Design review of the part built by this model. Coordinates are the model's own, in mm. Face numbers are marked on the shaded views. A direction names the side the tool comes from. Round coordinates to 2 decimals unless told otherwise and drop trailing zeros. Loops run counter-clockwise (first coordinate to the right, second up) from the corner with the lowest first, then second, coordinate; pieces in that order, holes last. Notation, with made-up numbers: (44.5, -8) -> (63.5, -8) arc R17 cw to (63.5, 20) -> close; hole circle Ø7 at (54.5, 44). An arc over 180 degrees is marked (long way). Answer as CSV lines item,"result". Start each with the question number.
(1) Take a section at B-B, the plane z = 95. Write out the cut boundary in (x, y), and give its area (3 significant figures).
(2) Take a section at C-C, the plane y = 79.5. Write out the cut boundary in (x, z), and give its area (3 significant figures).
(3) For P1, Ø5, axis at x = 25, z = -28.5, coming from the -Y side; P2, Ø6, axis at y = 97.5, z = 87, coming from the -X side, all flat-tipped, find the tip position at first contact; note any pin that passes through.
(4) Take a section at A-A, the plane x = -86. Write out the cut boundary in (y, z).
(5) To check wall thickness, follow line 1 (X direction, y = 5.5, z = -109.5); line 2 (X direction, y = -208.5, z = 106.5); line 3 (Z direction, x = -41, y = -149.5). State the ranges of each line that lie inside material, in increasing order. Write a range as from..to.
(6) Machinability: for the marked faces 4, 5 and 6, which of the approach directions +Z, -Z, +X, -X, +Y, -Y give a long, thin tool a straight path to every point of the face, cutting with its end or side? Answer none if there is none.
(7) Draft analysis for pull direction Z (two halves, no side actions). For the marked faces 1, 2 and 3, state which applies: +Z half, -Z half, draft (parallel to the pull), parting line (faces both ways), or undercut.
from build123d import *

# Parameters (mm, degrees)
SKETCH_2_W          = 22
SKETCH_2_H          = 50
EXTRUDE_1_DEPTH     = 3
EXTRUDE_2_DEPTH     = 20
CUT_EXTRUDE_1_DEPTH = 1
SKETCH_4_3_R        = 0.5
CUT_EXTRUDE_2_DEPTH = 2
SKETCH_5_W          = 22
SKETCH_5_H          = 50
EXTRUDE_3_DEPTH     = 3
SKETCH_8_R          = 0.5
CUT_EXTRUDE_3_DEPTH = 1.2
SKETCH_9_R          = 0.75
EXTRUDE_4_DEPTH     = 2
SCALE_1_SCALE       = 10


with BuildPart() as part:
    # Sketch 2 → Extrude 1 (new body)
    with BuildSketch(Plane.XY):
        Rectangle(SKETCH_2_W, SKETCH_2_H)
    extrude(amount=EXTRUDE_1_DEPTH)

    # Sketch 3 → Extrude 2 (add)
    with BuildSketch(Plane.XY.offset(3)):
        Polygon((-11, 20.230452477), (-10.5, 20.230452477), (-10.5, 24.5), (10.5, 24.5), (10.5, -24.5), (-10.5, -24.5), (-10.5, -19.769547523), (-11, -19.769547523), (-11, -25), (11, -25), (11, 25), (-11, 25), align=None)
    extrude(amount=EXTRUDE_2_DEPTH)

    # Sketch 4 → Cut-Extrude 1 (cut)
    with BuildSketch(Plane.XY.offset(3)):
        with BuildLine():
            ThreePointArc((4.079070714, 21.35), (6.553944448, 20.324873734), (7.579070714, 17.85))
            Line((7.579070714, 17.85), (7.579070714, -17.85))
            ThreePointArc((7.579070714, -17.85), (6.553944448, -20.324873734), (4.079070714, -21.35))
            Line((4.079070714, -21.35), (-3.920929286, -21.35))
            ThreePointArc((-3.920929286, -21.35), (-6.39580302, -20.324873734), (-7.420929286, -17.85))
            Line((-7.420929286, -17.85), (-7.420929286, 17.85))
            ThreePointArc((-7.420929286, 17.85), (-6.39580302, 20.324873734), (-3.920929286, 21.35))
            Line((-3.920929286, 21.35), (4.079070714, 21.35))
        make_face()
        with BuildLine():
            Line((-3.920929286, 20.35), (4.079070714, 20.35))
            ThreePointArc((4.079070714, 20.35), (5.846837667, 19.617766953), (6.579070714, 17.85))
            Line((6.579070714, 17.85), (6.579070714, -17.85))
            ThreePointArc((6.579070714, -17.85), (5.846837667, -19.617766953), (4.079070714, -20.35))
            Line((4.079070714, -20.35), (-3.920929286, -20.35))
            ThreePointArc((-3.920929286, -20.35), (-5.688696239, -19.617766953), (-6.420929286, -17.85))
            Line((-6.420929286, -17.85), (-6.420929286, 17.85))
            ThreePointArc((-6.420929286, 17.85), (-5.688696239, 19.617766953), (-3.920929286, 20.35))
        make_face(mode=Mode.SUBTRACT)
    extrude(amount=-CUT_EXTRUDE_1_DEPTH, mode=Mode.SUBTRACT)

    # Sketch 4_3 → Cut-Extrude 2 (cut)
    with BuildSketch(Plane.XY.offset(3)):
        with BuildLine():
            Line((6.079070714, 17.85), (6.079070714, -17.85))
            ThreePointArc((6.079070714, -17.85), (5.493284277, -19.264213562), (4.079070714, -19.85))
            Line((4.079070714, -19.85), (-3.920929286, -19.85))
            ThreePointArc((-3.920929286, -19.85), (-5.335142848, -19.264213562), (-5.920929286, -17.85))
            Line((-5.920929286, -17.85), (-5.920929286, 17.85))
            ThreePointArc((-5.920929286, 17.85), (-5.335142848, 19.264213562), (-3.920929286, 19.85))
            Line((-3.920929286, 19.85), (4.079070714, 19.85))
            ThreePointArc((4.079070714, 19.85), (5.493284277, 19.264213562), (6.079070714, 17.85))
        make_face()
        with Locations((-3.920929286, -17.85)):
            Circle(SKETCH_4_3_R, mode=Mode.SUBTRACT)
        with Locations((4.079070714, -17.85)):
            Circle(SKETCH_4_3_R, mode=Mode.SUBTRACT)
        with Locations((-3.920929286, 17.85)):
            Circle(SKETCH_4_3_R, mode=Mode.SUBTRACT)
        with Locations((4.079070714, 17.85)):
            Circle(SKETCH_4_3_R, mode=Mode.SUBTRACT)
        with BuildLine():
            Line((5.079070714, -16.731966011), (5.079070714, 16.731966011))
            ThreePointArc((5.079070714, 16.731966011), (3.018410542, 16.789339828), (2.961036725, 18.85))
            Line((2.961036725, 18.85), (-2.802895297, 18.85))
            ThreePointArc((-2.802895297, 18.85), (-2.860269114, 16.789339828), (-4.920929286, 16.731966011))
            Line((-4.920929286, 16.731966011), (-4.920929286, -16.731966011))
            ThreePointArc((-4.920929286, -16.731966011), (-2.860269114, -16.789339828), (-2.802895297, -18.85))
            Line((-2.802895297, -18.85), (2.961036725, -18.85))
            ThreePointArc((2.961036725, -18.85), (3.018410542, -16.789339828), (5.079070714, -16.731966011))
        make_face(mode=Mode.SUBTRACT)
    extrude(amount=-CUT_EXTRUDE_2_DEPTH, mode=Mode.SUBTRACT)

    # Sketch 5 → Extrude 3 (add)
    with BuildSketch(Plane.XY.offset(23)):
        Rectangle(SKETCH_5_W, SKETCH_5_H)
    extrude(amount=EXTRUDE_3_DEPTH)

    # Sketch 8 → Cut-Extrude 3 (cut)
    with BuildSketch(Plane.XY.offset(3)):
        with Locations((4.079070714, -17.85)):
            Circle(SKETCH_8_R)
        with Locations((4.079070714, 17.85)):
            Circle(SKETCH_8_R)
        with Locations((-3.920929286, 17.85)):
            Circle(SKETCH_8_R)
        with Locations((-3.920929286, -17.85)):
            Circle(SKETCH_8_R)
    extrude(amount=-CUT_EXTRUDE_3_DEPTH, mode=Mode.SUBTRACT)

    # Sketch 9 → Extrude 4 (add)
    with BuildSketch(Plane.XZ.offset(25)):
        with Locations(Location((0, 13, 0), (0, 0, 90))):
            Circle(SKETCH_9_R)
    extrude(amount=EXTRUDE_4_DEPTH)


with BuildPart() as part_1:
    # Scale 1: scaled about (0.58667368, -0.025272028, 13.505805339)
    add(part.part.scale(SCALE_1_SCALE).moved(Location((-5.28006312, 0.227448252, -121.552248051))))


solid = part_1.part
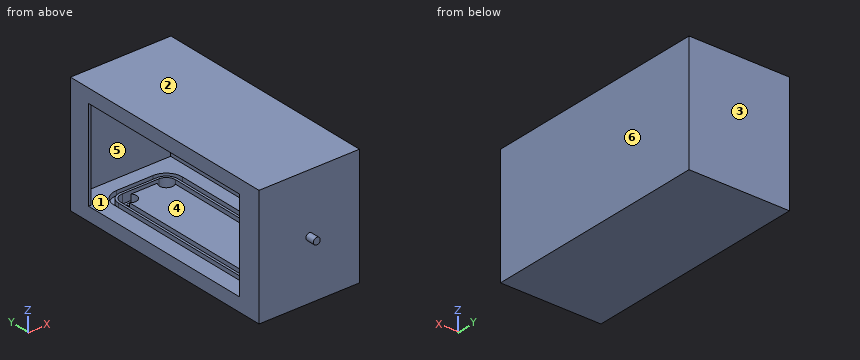
The answers:
1,outline,"(-115.28, -249.77) -> (104.72, -249.77) -> (104.72, 250.23) -> (-115.28, 250.23) -> (-115.28, 202.53) -> (-110.28, 202.53) -> (-110.28, 245.23) -> (99.72, 245.23) -> (99.72, -244.77) -> (-110.28, -244.77) -> (-110.28, -197.47) -> (-115.28, -197.47) -> close"
1,area,"5,100 mm²"
2,outline,"(-115.28, -121.55) -> (104.72, -121.55) -> (104.72, 138.45) -> (-115.28, 138.45) -> (-115.28, 108.45) -> (99.72, 108.45) -> (99.72, -91.55) -> (70.51, -91.55) -> (70.51, -101.55) -> (60.51, -101.55) -> (60.51, -91.55) -> (55.51, -91.55) -> (55.51, -111.55) -> (45.51, -111.55) -> (45.51, -91.55) -> (-54.49, -91.55) -> (-54.49, -111.55) -> (-64.49, -111.55) -> (-64.49, -91.55) -> (-69.49, -91.55) -> (-69.49, -101.55) -> (-79.49, -101.55) -> (-79.49, -91.55) -> (-115.28, -91.55) -> close"
2,area,"13,600 mm²"
3,P1,"y = -249.77"
3,P2,"x = 99.72"
4,outline,"(-249.77, -121.55) -> (250.23, -121.55) -> (250.23, 138.45) -> (-249.77, 138.45) -> close; hole (-244.77, -91.55) -> (245.23, -91.55) -> (245.23, 108.45) -> (-244.77, 108.45) -> close"
5,line 1,"-115.28..-64.49, -54.49..45.51, 55.51..104.72"
5,line 2,"-115.28..-110.28, 99.72..104.72"
5,line 3,"-121.55..-91.55, 108.45..138.45"
6,face 4,"-X"
6,face 5,"none"
6,face 6,"+Z, -Z, +X, +Y, -Y"
7,face 1,"undercut"
7,face 2,"+Z half"
7,face 3,"draft"
